Autodesk Inventor part; units mm, degrees
ref_plane "YZ Plane" through (0, 0, 0) normal (1, 0, 0) x (0, 1, 0)
ref_plane "XZ Plane" through (0, 0, 0) normal (0, 1, 0) x (-1, 0, 0)
ref_plane "XY Plane" through (0, 0, 0) normal (0, 0, 1) x (1, 0, 0)
sketch "Esquisse1" plane through (0, 0, 0) normal (1, 0, 0) x (0, 1, 0)
  arc A0 (13, -11.5) -> (13, 11.5) centre (13, 0) ccw
  line L0 (-13, 11.5) -> (13, 11.5)
  line L1 (13, 11.5) -> (13, -11.5) construction
  line L2 (13, -11.5) -> (-13, -11.5)
  line L3 (-13, -11.5) -> (-13, 11.5)
  line L4 (-13, 11.5) -> (13, -11.5) construction
  line L5 (13, 11.5) -> (-13, -11.5) construction
  line L6 (-3, 11.5) -> (-3, -11.5)
  circle A1 centre (13, 0) radius 11.5 construction
  point P0 (0, 0)
  point P1 (0, 0)
  dimension "d1" = 23
  dimension "d2" = 16
  dimension "d3" = 10
extrude "Extrusion1" add sketch "Esquisse1" along normal blind 8
extrude "Extrusion2" add sketch "Esquisse1" against normal blind 1.5 contours L2 L6 L0 A0
sketch "Esquisse3" plane through (8, 0, 0) normal (1, 0, 0) x (0, 0, -1)
  arc A0 (11.5, 13) -> (-11.5, 13) centre (0, 13) ccw
  point P0 (0, 0)
  point P1 (0, 13)
hole "Perçage1" at (8, 13, 0) direction (-1, 0, 0) diameter 10 end through all counterbore diameter 15 counterbore depth 5
sketch "Esquisse4" plane through (-1.5, 0, 0) normal (-1, 0, 0) x (0, 0, 1)
  circle A0 centre (0, 13) radius 5
  circle A1 centre (0, 13) radius 8.75 construction
  circle A2 centre (0, 13) radius 7.5
  line L0 (8.75, 13) -> (-8.75, 13)
  point P0 (0, 0)
  dimension "d15" = 17.5
hole "Perçage2" at (-1.5, 13, -8.75) at (-1.5, 13, 8.75) direction (1, 0, 0) diameter 3.2 depth 4
sketch "Esquisse5" plane through (8, 0, 0) normal (1, 0, 0) x (0, 0, -1)
  line L0 (18, 3) -> (-18, 3)
  line L1 (-18, 3) -> (-18, -3)
  line L2 (-18, -3) -> (18, -3)
  line L3 (18, -3) -> (18, 3)
  line L4 (18, 3) -> (-18, -3) construction
  line L5 (-18, 3) -> (18, -3) construction
  line L6 (11.5, -13) -> (11.5, 13) construction
  line L7 (11.5, -3) -> (-11.5, -3)
  point P0 (0, 0)
  dimension "d23" = 6.5
extrude "Extrusion3" add sketch "Esquisse5" against normal blind 28
fillet "Congé1" radius 2 10 edges at (8, 0, 18) (-20, 0, 18) (3.25, 3, 11.5) (4, -3, 11.5) (4, -3, -11.5) (8, 0, -18) (3.25, 3, -11.5) (-20, 0, -18) (4, -13, -11.5) (4, -13, 11.5)
sketch "Esquisse6" plane through (8, 3, 16) normal (0, 1, 0) x (1, 0, 0)
  line L0 (-18, 29.8634) -> (-18, 2.1366) construction
  line L1 (-9.5, 11) -> (-9.5, 21)
  line L2 (-5, 11) -> (-5, 21)
  line L3 (-11.5, 29.5) -> (-11.5, 2.5)
  line L4 (-11.5, 16) -> (-28, 16) construction
  line L5 (-28, 32) -> (-28, 0)
  point P0 (-8, 16)
  point P1 (-18, 16)
  dimension "d27" = 10
hole "Perçage3" at (-10, 3, -13.8634) at (-10, 3, 13.8634) direction (0, -1, 0) diameter 4.2 end through all countersink diameter 6 countersink angle 90
sketch "Esquisse7" plane through (-1.5, 0, 0) normal (-1, 0, 0) x (0, 0, 1)
  circle A0 centre (0, 13) radius 11.75
  arc A1 (11.5, 13) -> (-11.5, 13) centre (0, 13) ccw construction
  point P0 (0, 0)
  dimension "d36" = 23.5
extrude "Extrusion4" cut sketch "Esquisse7" along normal through all
properties part number "support_codeur"
Build history of the part. All positions in model axes, mm. A direction names the side the tool comes from. Give positions to 0.01 mm unless a question says otherwise; leave off trailing zeros. Order: outer loops, then holes, each group sorted by start corner. A loop starts at its lowest first (then second) coordinate and runs counter-clockwise, first axis right, second up. Notation, with made-up numbers: M 29,34 L 84,34 A23 ccw 84,67 Z; hole C 81,1 d6. An arc over 180 degrees is marked long. Use one line per item in the form item = value.
1) Saw through at D-D (y = 17.5). Give the cut face in (x, z), plus the area to 3 significant figures.
Calculated:
outline = M -1.5,-10.58 L 8,-10.58 L 8,-6 L 3,-6 L 3,-2.18 L -1.5,-2.18 Z; M -1.5,2.18 L 3,2.18 L 3,6 L 8,6 L 8,10.58 L -1.5,10.58 Z
area = 121 mm2
2) Two-plate mould, pull along X, no slides. Class faces 1 (the face through (7.43, 0.04, -17.4)), 2 (the face through (3.32, 3.57, 12.1)), 3 (the face through (-20, 0, 0)), 4 (the face through (-10.631, -0.486, 15.866)): released by +X, released by -X, zero draft, split by the parting line, or undercut.
Calculated:
face_1 = released by +X
face_2 = zero draft
face_3 = released by -X
face_4 = undercut
3) Tool access for faces 5 (the face through (3, 18, -2)), 6 (the face through (3, 9, 11.5)), 7 (the face through (-8.9, 3, -10.9)): list every direction of +Z, -Z, +X, -X, +Y, -Y with a clear straight run to the whole face (end or side of a thin tool).
Calculated:
face_5 = +X
face_6 = +Z, +X, -X, +Y
face_7 = -Z, -X, +Y
4) Saw through at A-A (x = 0.5). Give the cut face in (y, z).
Calculated:
outline = M -13,-9.5 A2 ccw -11,-11.5 L -5,-11.5 A2 cw -3,-13.5 L -3,-18 L 3,-18 L 3,-13.5 A2 cw 5,-11.5 L 13,-11.5 A11.5 ccw 13,11.5 L 5,11.5 A2 cw 3,13.5 L 3,18 L -3,18 L -3,13.5 A2 cw -5,11.5 L -11,11.5 A2 ccw -13,9.5 Z; hole C 13,0 d10; hole C 13,-8.75 d3.2; hole C 13,8.75 d3.2
5) Probe probe 1 along Z at (x, y) = (-10, -1.65); probe 2 along Z at (x, y) = (0, 13); probe 3 along Y at (x, z) = (-16.5, -10). List the from-to ranges inside material, lowest first.
Calculated:
probe_1 = -18 to -15.96, -11.76 to 11.76, 15.96 to 18
probe_2 = -11.5 to -10.35, -7.15 to -5, 5 to 7.15, 10.35 to 11.5
probe_3 = -3 to 3
6) Saw through at C-C (x = -10). Give the cut face in (y, z).
Calculated:
outline = M -3,-18 L 3,-18 L 3,-16.86 L 2.1,-15.96 L -3,-15.96 Z; M -3,-11.76 L 2.1,-11.76 L 3,-10.86 L 3,-6.17 A11.75 cw 3,6.17 L 3,10.86 L 2.1,11.76 L -3,11.76 Z; M -3,15.96 L 2.1,15.96 L 3,16.86 L 3,18 L -3,18 Z
7) Saw through at B-B (z = 1.5). Give the cut face in (x, y).
Calculated:
outline = M -20,-3 L 0,-3 L 0,-13 L 8,-13 L 8,5.65 L 3,5.65 L 3,8.23 L -1.5,8.23 L -1.5,1.35 L -20,1.35 Z; M -1.5,17.77 L 3,17.77 L 3,20.35 L 8,20.35 L 8,24.4 L -1.5,24.4 Z
8) Drop flat-ended pins along their axis: pin 1 (6.5 mm diameter, centred on x = 1, y = 9, fed in from +Z); pin 2 (2.5 mm diameter, centred on y = 12.5, z = 9.5, fed in from -X); pin 3 (4 mm diameter, centred on x = -16.5, z = 12.5, fed in from +Y). Give the stop position or say it passes through.
Calculated:
pin_1 = 11.5
pin_2 = -1.5
pin_3 = 3
